```python
from build123d import *

# Parameters (mm, degrees)
BOSS_EXTRUDE1_DEPTH = 25
CUT_EXTRUDE1_REACH  = 1305.476


with BuildPart() as part:
    # Sketch1 → Boss-Extrude1 (new body)
    with BuildSketch(Plane(origin=(0, 0, 0), x_dir=(0, 0, -1), z_dir=(1, 0, 0))):
        with BuildLine():
            Line((0, 50), (0, 1195))
            Line((0, 1195), (200, 1195))
            Line((200, 1195), (517.768948114, 167.216058445))
            ThreePointArc((517.768948114, 167.216058445), (519.439090838, 159.915268109), (520, 152.446915067))
            Line((520, 152.446915067), (520, 0))
            Line((520, 0), (50, 0))
            ThreePointArc((50, 0), (35.355339059, 35.355339059), (0, 50))
        make_face()
    extrude(amount=-BOSS_EXTRUDE1_DEPTH)

    # Sketch2 → Cut-Extrude1 (cut, up to next)
    with BuildSketch(Plane(origin=(0, 0, 0), x_dir=(0, 0, -1), z_dir=(1, 0, 0)), mode=Mode.PRIVATE) as cut_extrude1_sk1:
        with BuildLine():
            Line((90, 120), (90, 420))
            ThreePointArc((90, 420), (95.857864376, 434.142135624), (110, 440))
            Line((110, 440), (334.943019945, 440))
            ThreePointArc((334.943019945, 440), (346.814137267, 436.095855787), (354.05059919, 425.907657351))
            Line((354.05059919, 425.907657351), (439.107579245, 150.801487485))
            ThreePointArc((439.107579245, 150.801487485), (439.775636335, 147.881171351), (440, 144.893830134))
            Line((440, 144.893830134), (440, 120))
            ThreePointArc((440, 120), (434.142135624, 105.857864376), (420, 100))
            Line((420, 100), (110, 100))
            ThreePointArc((110, 100), (95.857864376, 105.857864376), (90, 120))
        make_face()
    cut_extrude1_tool1 = extrude(cut_extrude1_sk1.sketch, amount=-CUT_EXTRUDE1_REACH, mode=Mode.PRIVATE) & part.part
    # Sketch2 → Cut-Extrude1 (cut, up to next)
    with BuildSketch(Plane(origin=(0, 0, 0), x_dir=(0, 0, -1), z_dir=(1, 0, 0)), mode=Mode.PRIVATE) as cut_extrude1_sk2:
        with BuildLine():
            Line((90, 590), (90, 1075))
            ThreePointArc((90, 1075), (95.857864376, 1089.142135624), (110, 1095))
            Line((110, 1095), (132.43094265, 1095))
            ThreePointArc((132.43094265, 1095), (144.302059973, 1091.095855787), (151.538521896, 1080.907657351))
            Line((151.538521896, 1080.907657351), (301.490212717, 595.907657351))
            ThreePointArc((301.490212717, 595.907657351), (298.478489258, 578.128882677), (282.382633471, 570))
            Line((282.382633471, 570), (110, 570))
            ThreePointArc((110, 570), (95.857864376, 575.857864376), (90, 590))
        make_face()
    cut_extrude1_tool2 = extrude(cut_extrude1_sk2.sketch, amount=-CUT_EXTRUDE1_REACH, mode=Mode.PRIVATE) & part.part
    add(cut_extrude1_tool1.solids().sort_by_distance((0, 260.991144, -246.99454))[0], mode=Mode.SUBTRACT)
    add(cut_extrude1_tool2.solids().sort_by_distance((0, 781.346957, -166.978745))[0], mode=Mode.SUBTRACT)


solid = part.part
```
Work out the finished part from the listing and answer in its coordinate system (mm). A direction names the side the tool comes from. Give positions to 0.01 mm unless a question says otherwise; leave off trailing zeros. Order: outer loops, then holes, each group sorted by start corner. A loop starts at its lowest first (then second) coordinate and runs counter-clockwise, first axis right, second up.
1. For faces 1 (the flat face through (-12, 570, -197)), 2 (the flat face through (-12, 614, 0)), determine the directions among +Z, -Z, +X, -X, +Y, -Y from which every point of the face is accessible in a straight line to the end or side of a thin tool.
Result sheet:
face 1: +X, -X
face 2: +Z, +X, -X, +Y, -Y
2. Section D-D, the plane y = 389 is taken. Determine the outline of the cut face in (x, z), and give its area (3 significant figures).
Result sheet:
outline: (-25, -449.2) - (0, -449.2) - (0, -365.46) - (-25, -365.46) - close; (-25, -90) - (0, -90) - (0, 0) - (-25, 0) - close
area: 4,340 mm2
3. Section B-B, the plane x = -5 is taken. Determine the outline of the cut face in (y, z), and give its area (3 significant figures).
Result sheet:
outline: (0, -520) - (152.45, -520) arc R50 ccw to (167.22, -517.77) - (1195, -200) - (1195, 0) - (50, 0) arc R50 cw to (0, -50) - close; hole (100, -420) arc R20 ccw to (120, -440) - (144.89, -440) arc R20 ccw to (150.8, -439.11) - (425.91, -354.05) arc R20 ccw to (440, -334.94) - (440, -110) arc R20 ccw to (420, -90) - (120, -90) arc R20 ccw to (100, -110) - close; hole (570, -282.38) arc R20 ccw to (595.91, -301.49) - (1080.91, -151.54) arc R20 ccw to (1095, -132.43) - (1095, -110) arc R20 ccw to (1075, -90) - (590, -90) arc R20 ccw to (570, -110) - close
area: 276,000 mm2
4. Section A-A, the plane z = -391.5 is taken. Determine the outline of the cut face in (x, y).
Result sheet:
outline: (-25, 0) - (0, 0) - (0, 100) - (-25, 100) - close; (-25, 304.78) - (0, 304.78) - (0, 575.62) - (-25, 575.62) - close
5. The mould has two halves that part along Y. Classify faces 3 (the flat face through (-12, 100, -267)), 4 (the flat face through (-12.325, 290.28, -395.984)), 5 (the cylindrical face through (-12.325, 34.964, -35.742)), 6 (the flat face through (0, 473, -206)): released by +Y, released by -Y, zero draft, split by the parting line, or undercut.
Result sheet:
face 3: undercut
face 4: undercut
face 5: released by -Y
face 6: zero draft
6. Each of these flat-tipped pins is pushed along its axis until it touches: P1, Ø2, axis at y = 247.5, z = -82.5, coming from the +X side; P2, Ø8, axis at x = -8, y = 648.5, coming from the -Z side. Where does it stop, or does it pass through?
Result sheet:
P1: stops at x = 0
P2: stops at z = -370.2
7. Section C-C, the plane z = -178 is taken. Determine the outline of the cut face in (x, y).
Result sheet:
outline: (-25, 0) - (0, 0) - (0, 100) - (-25, 100) - close; (-25, 440) - (0, 440) - (0, 570) - (-25, 570) - close; (-25, 995.32) - (0, 995.32) - (0, 1195) - (-25, 1195) - close
8. Straight lines are drawn through the part: L1, parallel to Z at x = -10.75, y = 1006; L2, parallel to Z at x = -10.25, y = 839; L3, parallel to Z at x = -22.5, y = 484.5. For each, find the intervals that lie inside material, in ascending order.
Result sheet:
L1: z = -258.43 to -174.7, -90 to 0
L2: z = -310.07 to -226.33, -90 to 0
L3: z = -419.67 to 0
